Work out the finished part from the listing and answer in its coordinate system (mm). Face numbers are marked on the shaded views. A direction names the side the tool comes from. Give positions to 0.01 mm unless a question says otherwise; leave off trailing zeros. Order: outer loops, then holes, each group sorted by start corner. A loop starts at its lowest first (then second) coordinate and runs counter-clockwise, first axis right, second up. Notation, with made-up numbers: (52, 9) -> (62, 9) arc R19 cw to (62, 44) -> close; hole circle Ø5 at (65.5, 84). An arc over 180 degrees is marked (long way). Answer as CSV lines item,"result". Start each with the question number.
1. Find the intervals of material crossed by L1, parallel to Y at x = 15, z = 4; L2, parallel to Z at x = 48.5, y = 13; L3, parallel to Z at x = 7.5, y = 3, in increasing order.
2. A cutting plane is placed at D-D (z = -6). Give the vertices of the cut face in (x, y).
3. A cutting plane is placed at B-B (z = 1.5). Give the vertices of the cut face in (x, y).
4. A cutting plane is placed at A-A (x = 44). Give the vertices of the cut face in (y, z), then the cut area to 3 significant figures.
5. Flat-ended cylindrical pins translate along their axes: pin 1 (3 mm diameter, centred on y = 6, z = 6.5, fed in from +X); pin 2 (11 mm diameter, centred on y = 37, z = 13.5, fed in from -X); pin 3 (10 mm diameter, centred on x = 6.5, z = 3.5, fed in from -Y); pin 4 (5 mm diameter, centred on x = 9, z = 5, fed in from +Y). Find the tip coordinate at first contact, or state that the pin passes through.
6. For the marked faces 1, 2 and 3, determine the directions among +Z, -Z, +X, -X, +Y, -Y from which every point of the face is accessible in a straight line to the end or side of a thin tool.
7. For a pull along Y with two mould halves and no side action, classify the marked faces 4, 5 and 6 as released by +Y, released by -Y, zero draft, split by the parting line, or undercut.
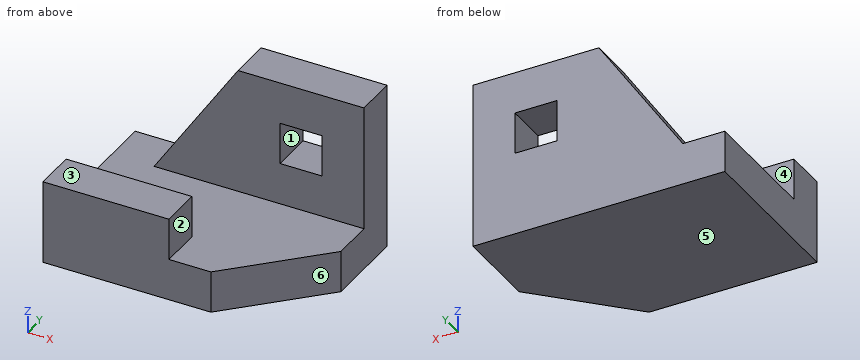
from build123d import *

# Parameters (mm, degrees)
F0_W     = 30
F0_H     = 10
F0_W_2   = 50
F1_DEPTH = 10
F2_DEPTH = 10
F3_DEPTH = 30
F4_W     = 10
F4_H     = 10
F5_DEPTH = 10
F6_SIZE2 = 29.99999
F6_SIZE  = 19.99999


# Not quite as in the source:
# - a fillet or chamfer is up to 0.001 mm smaller than in the source, because OpenCascade refuses the exact size


with BuildPart() as f1:
    # F0 (on Top) → F1 (new body)
    with BuildSketch(Plane.XY):
        with Locations((15, 5)):
            Rectangle(F0_W, F0_H)
        with Locations((35, 35)):
            Rectangle(F0_W_2, F0_H)
        Polygon((30, 10), (30, 0), (40, 0), (60, 20), (60, 30), (10, 30), (10, 40), (0, 40), (0, 10), align=None)
    extrude(amount=-F1_DEPTH)

    # F0 (on Top) → F2 (join)
    with BuildSketch(Plane.XY):
        with Locations((15, 5)):
            Rectangle(F0_W, F0_H)
    extrude(amount=F2_DEPTH)

    # F0 (on Top) → F3 (join)
    with BuildSketch(Plane.XY):
        with Locations((35, 35)):
            Rectangle(F0_W_2, F0_H)
    extrude(amount=F3_DEPTH)

    # F4 (on face) → F5 (cut)
    with BuildSketch(Plane(origin=(0, 40, 0), x_dir=(-1, 0, 0), z_dir=(0, 1, 0))):
        with Locations((-45, 15)):
            Rectangle(F4_W, F4_H)
    extrude(amount=-F5_DEPTH, mode=Mode.SUBTRACT)

    # F6 (size 20 and 30 in the source; OpenCascade refuses exactly that, so slightly less here)
    f6_edges = [f1.edges().sort_by_distance(p)[0] for p in [
        (10, 35, 30),
    ]]
    f6_side = f1.faces().sort_by_distance((35, 35, 30))[0]
    chamfer(f6_edges, length=F6_SIZE, length2=F6_SIZE2, reference=f6_side)


solid = f1.part
Answer sheet:
1,L1,"y = 0 to 10, 30 to 40"
1,L2,"z = -10 to 0"
1,L3,"z = -10 to 10"
2,outline,"(0, 0) -> (40, 0) -> (60, 20) -> (60, 40) -> (0, 40) -> close"
3,outline,"(0, 0) -> (30, 0) -> (30, 10) -> (0, 10) -> close; (11, 30) -> (60, 30) -> (60, 40) -> (11, 40) -> close"
4,outline,"(4, -10) -> (40, -10) -> (40, 10) -> (30, 10) -> (30, 0) -> (4, 0) -> close; (30, 20) -> (40, 20) -> (40, 30) -> (30, 30) -> close"
4,area,"560 mm^2"
5,pin 1,"stops at x = 30"
5,pin 2,"stops at x = 15.33"
5,pin 3,"stops at y = 0"
5,pin 4,"stops at y = 10"
6,face 1,"+Y, -Y"
6,face 2,"+Z, +X, -Y"
6,face 3,"+Z, +X, -X, -Y"
7,face 4,"undercut"
7,face 5,"zero draft"
7,face 6,"released by -Y"
